Can you work these out from the drawing? Everything is in mm from the part's minimum corner. A direction names the side the tool comes from. Round coordinates to 2 decimals unless told otherwise and drop trailing zeros. Order: outer loops, then holes, each group sorted by start corner. A loop starts at its lowest first (then second) coordinate and runs counter-clockwise, first axis right, second up. Notation, with made-up numbers: (63.5, 23) - (106.5, 23) arc R11 cw to (106.5, 31) - close; hole circle Ø5 at (17, -33). An arc over 180 degrees is marked (long way). Write item = value, one per line.
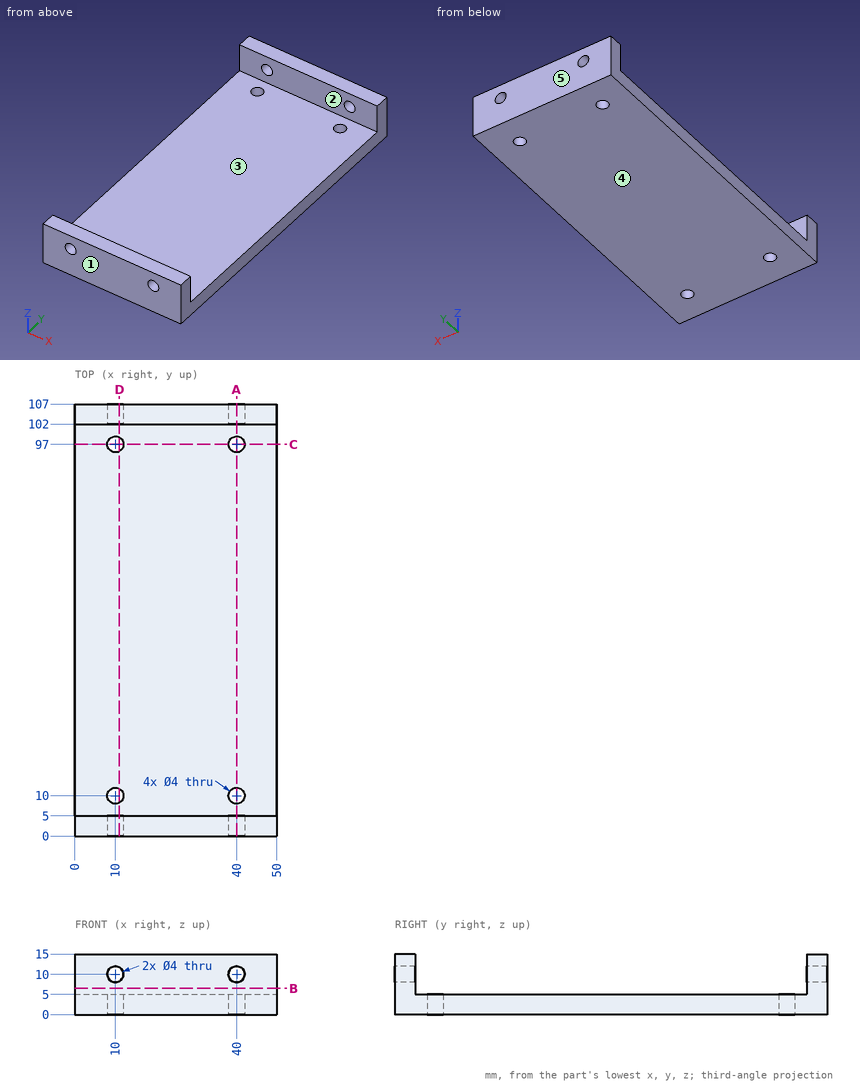
(1) Will these pins go through, and if not, where does the flat tip stop? P1, Ø4, axis at x = 40.5, z = 4.5, coming from the -Y side; P2, Ø3, axis at x = 19.5, y = 77, coming from the +Z side.
Computed:
P1 = 0
P2 = 5
(2) If we section it at D-D (x = 11): Write out the boundary of the cut face in (y, z), plus the area to 3 significant figures.
Computed:
outline = (0, 0) - (8.27, 0) - (8.27, 5) - (5, 5) - (5, 8.27) - (0, 8.27) - close; (0, 11.73) - (5, 11.73) - (5, 15) - (0, 15) - close; (11.73, 0) - (95.27, 0) - (95.27, 5) - (11.73, 5) - close; (98.73, 0) - (107, 0) - (107, 8.27) - (102, 8.27) - (102, 5) - (98.73, 5) - close; (102, 11.73) - (107, 11.73) - (107, 15) - (102, 15) - close
area = 566 mm^2
(3) If we section it at C-C (y = 97): Write out the boundary of the cut face in (x, z), plus the area to 3 significant figures.
Computed:
outline = (0, 0) - (8, 0) - (8, 5) - (0, 5) - close; (12, 0) - (38, 0) - (38, 5) - (12, 5) - close; (42, 0) - (50, 0) - (50, 5) - (42, 5) - close
area = 210 mm^2
(4) If we section it at B-B (z = 6.5): Write out the boundary of the cut face in (x, y).
Computed:
outline = (0, 0) - (50, 0) - (50, 5) - (0, 5) - close; (0, 102) - (50, 102) - (50, 107) - (0, 107) - close
(5) Thinking about a two-plate mould opening in Y: for the marked faces 3, 4 and 5, which applies, +Y half, -Y half, draft (parallel to the pull), parting line (faces both ways), or undercut?
Computed:
face_3 = undercut
face_4 = draft
face_5 = +Y half
(6) If we section it at A-A (x = 40): Write out the boundary of the cut face in (y, z).
Computed:
outline = (0, 0) - (8, 0) - (8, 5) - (5, 5) - (5, 8) - (0, 8) - close; (0, 12) - (5, 12) - (5, 15) - (0, 15) - close; (12, 0) - (95, 0) - (95, 5) - (12, 5) - close; (99, 0) - (107, 0) - (107, 8) - (102, 8) - (102, 5) - (99, 5) - close; (102, 12) - (107, 12) - (107, 15) - (102, 15) - close
(7) If I drill on line 1 (X direction, y = 105.3, z = 10); line 2 (Y direction, x = 10, z = 3.9); line 3 (Y direction, x = 16, z = 10.75), over which ranges is the centre line in solid material (lowest first)? Write a range as from..to.
Computed:
line_1 = 0..8, 12..38, 42..50
line_2 = 0..8, 12..95, 99..107
line_3 = 0..5, 102..107
(8) On a 3-axis mill with a long thin cutter (end or side, diameter ignored), from which of +Z, -Z, +X, -X, +Y, -Y can I reach the whole of each face in a straight line? I mean the marked faces 1 and 2. Say none if no direction works.
Computed:
face_1 = +Z, -Z, +X, -X, -Y
face_2 = +Z, +X, -X
